Read the model definition and answer for the solid it produces. Units are mm, in the model's axes. A direction names the side the tool comes from. Give positions to 0.01 mm unless a question says otherwise; leave off trailing zeros. Loops run counter-clockwise (first coordinate to the right, second up) from the corner with the lowest first, then second, coordinate; pieces in that order, holes last.
(1) Find section B-B, the plane z = -14.5. Write down the section's boundary in (x, y).
(2) Which of the six approach directions +Z, -Z, +X, -X, +Y, -Y give full straight-line access (tool end or side, diameter ignored) to faces 1 (the face through (-2, 636, 21.438)), 2 (the face through (0, -10, 24.613)), 3 (the face through (-18.263, -8, -3)), 4 (the face through (-2, -634, 21.438))?
(3) Each of these flat-tipped pins is pushed along its axis until it touches: P1, Ø5, axis at y = 610.5, z = 20.5, coming from the -X side; P2, Ø25, axis at x = -8, y = -651.5, coming from the +Z side; P3, Ø2.5, axis at x = 4, z = 23, coming from the -Y side; P4, Ø5.5, axis at x = -7.94, y = 596.9, coming from the -Z side. Where does it stop, or does it pass through?
(4) Straight lines are drawn through the part: probe 1 along X at (y, z) = (596.9, 19.2); probe 2 along X at (y, z) = (86.5, -15); probe 3 along Z at (x, y) = (12, 153). For each, find the intervals that lie inside material, in ascending order.
(5) Find section A-A, the plane y = -235. Write down the section's boundary in (x, z).
```python
from build123d import *

# Parameters (mm, degrees)
F1_DEPTH = 685.8
F2_W     = 30.95625
F2_H     = 101.6
F2_R     = 3.175
F3_DEPTH = 3.175
F4_DEPTH = 49.2262
F5_D     = 6.35


with BuildPart() as f1:
    # F0 (on Front) → F1 (new body, symmetric)
    with BuildSketch(Plane.XZ):
        Polygon((-24.6126, -24.6126), (-18.2626, -24.6126), (-18.2626, 18.2626), (24.6126, 18.2626), (24.6126, 24.6126), (-24.6126, 24.6126), align=None)
    extrude(amount=F1_DEPTH, both=True)

    # F2 (on face) → F3 (cut)
    with BuildSketch(Plane.XY.offset(24.6126)):
        with Locations((-1.990725, -635)):
            Rectangle(F2_W, F2_H)
        with Locations((-7.94385, -673.1)):
            Circle(F2_R, mode=Mode.SUBTRACT)
        with Locations((-7.94385, -622.3)):
            Circle(F2_R, mode=Mode.SUBTRACT)
        with Locations((3.9624, -647.7)):
            Circle(F2_R, mode=Mode.SUBTRACT)
        with Locations((3.9624, -596.9)):
            Circle(F2_R, mode=Mode.SUBTRACT)
        with Locations((-1.990725, 635)):
            Rectangle(F2_W, F2_H)
        with Locations((-7.94385, 596.9)):
            Circle(F2_R, mode=Mode.SUBTRACT)
        with Locations((-7.94385, 647.7)):
            Circle(F2_R, mode=Mode.SUBTRACT)
        with Locations((3.9624, 622.3)):
            Circle(F2_R, mode=Mode.SUBTRACT)
        with Locations((3.9624, 673.1)):
            Circle(F2_R, mode=Mode.SUBTRACT)
    extrude(amount=-F3_DEPTH, mode=Mode.SUBTRACT)

    # F2 (on face) → F4 (cut, through all)
    with BuildSketch(Plane.XY.offset(24.6126)):
        Polygon((-24.6126, 685.8), (-24.6126, 577.85), (-17.46885, 577.85), (-17.46885, 584.2), (-17.46885, 685.8), align=None)
        Polygon((-24.6126, -577.85), (-24.6126, -685.8), (-17.46885, -685.8), (-17.46885, -584.2), (-17.46885, -577.85), align=None)
    extrude(amount=-F4_DEPTH, mode=Mode.SUBTRACT)

    # F5 (through all)
    with Locations(Plane.XY.offset(24.6126)):
        with Locations((-7.94385, -673.1), (3.9624, -647.7), (-7.94385, -622.3), (3.9624, -596.9), (-7.94385, 647.7), (3.9624, 673.1), (3.9624, 622.3), (-7.94385, 596.9)):
            Hole(F5_D / 2)


solid = f1.part
```
Entries:
1. outline: (-24.61, -577.85) - (-18.26, -577.85) - (-18.26, 577.85) - (-24.61, 577.85) - close
2. face 1: +Z, -X, +Y
2. face 2: +Z, +X, -X, +Y, -Y
2. face 3: -Z, +X, +Y, -Y
2. face 4: +Z, -X, -Y
3. P1: stops at x = -17.47
3. P2: stops at z = 21.44
3. P3: stops at y = -584.2
3. P4: passes through
4. probe 1: x = -17.47 to -11.12, -4.77 to 24.61
4. probe 2: x = -24.61 to -18.26
4. probe 3: z = 18.26 to 24.61
5. outline: (-24.61, -24.61) - (-18.26, -24.61) - (-18.26, 18.26) - (24.61, 18.26) - (24.61, 24.61) - (-24.61, 24.61) - close
